Can you work these out from the model? Positions are in its coordinate system, mm. A direction names the side the tool comes from. Coordinates: 2 decimals unless noted, no trailing zeros. Order: outer loops, then holes, each group sorted by start corner. A loop starts at its lowest first (then second) coordinate and runs counter-clockwise, first axis right, second up. Notation, with made-up numbers: (-35, 33.5) -> (11, 33.5) arc R24 ccw to (11, 54.5) -> close; hole circle Ø1 at (86.25, 11.25). An arc over 180 degrees is marked (long way). Return JSON: item names as keys, results as strings. Group by question number.
1) For faces 1 (the flat face through (2, 50.8, 2)), 2 (the flat face through (2, 25.4, -46)), 3 (the flat face through (2, 50.8, -46)), 4 (the flat face through (2, 34.2, -22)), which set-ups out of +Z, -Z, +X, -X, +Y, -Y let a thin tool reach every point of the face, with its end or its side?
2) If we section it at A-A, the plane y = 66.7: Please give me the cut outline in (x, z) (3 decimals), then the cut area to 3 significant figures.
3) If we section it at D-D, the plane y = 10.5: Please give me the cut outline in (x, z) (3 decimals), then the cut area to 3 significant figures.
4) Thinking about a two-plate mould opening in Y: for faces 5 (the flat face through (2, 25.4, 2)), 6 (the flat face through (2, 49, -16.225)), 7 (the flat face through (2, 13, -44.45)), which applies, +Y half, -Y half, draft (parallel to the pull), parting line (faces both ways), or undercut?
5) If we section it at B-B, the plane x = 1.25: Please give me the cut outline in (y, z) (3 decimals), then the cut area to 3 significant figures.
6) If I drill on probe 1 along Y at (x, z) = (1.65, -27.5) (3 decimals); probe 2 along Z at (x, y) = (2.1, 52.5) (3 decimals); probe 3 along Z at (x, y) = (1.3, 48) (3 decimals), over which ranges is the centre line in solid material (lowest first)? Write a range as from..to.
7) If we section it at C-C, the plane y = 31.7: Please give me the cut outline in (x, z) (3 decimals).
8) For pin 1 (1.6 mm diameter, centred on x = 1.5, y = 74, fed in from +Z); pin 2 (12 mm diameter, centred on y = 46, z = -41, fed in from -X); pin 3 (1.6 mm diameter, centred on x = 1.5, z = 2, fed in from +Y); pin 4 (1.6 mm diameter, centred on x = 1, z = 2, fed in from -Y), each with a flat end and sliding along its axis, tell me the tip position at first contact or that it passes through.
Autodesk Inventor part; units mm, degrees
ref_plane "YZ Plane" through (0, 0, 0) normal (1, 0, 0) x (0, 1, 0)
ref_plane "XZ Plane" through (0, 0, 0) normal (0, 1, 0) x (-1, 0, 0)
ref_plane "XY Plane" through (0, 0, 0) normal (0, 0, 1) x (1, 0, 0)
sketch "Sketch1" plane through (0, 0, 0) normal (1, 0, 0) x (0, 1, 0)
  line L0 (0, 0) -> (76.2, 0)
  line L1 (76.2, 0) -> (76.2, -44.45)
  line L2 (76.2, -44.45) -> (0, -44.45)
  line L3 (0, -44.45) -> (0, 0)
  dimension "d0" = 76.2
  dimension "d1" = 44.45
extrude "Extrusion1" add sketch "Sketch1" along normal blind 3.175
sketch "Sketch2" plane through (3.175, 0, 0) normal (1, 0, 0) x (0, 0, -1)
  line L0 (44.45, 76.2) -> (0, 76.2)
  line L1 (13.7583, 76.2) -> (30.6917, 76.2)
  line L2 (30.6917, 76.2) -> (30.6917, 73.025)
  line L3 (30.6917, 73.025) -> (13.7583, 73.025)
  line L4 (13.7583, 73.025) -> (13.7583, 76.2)
  line L5 (0, 76.2) -> (0, 0)
  dimension "d4" = 16.9333
  dimension "d5" = 3.175
  dimension "d8" = 13.7583
extrude "Extrusion2" cut sketch "Sketch2" against normal blind 3.175
sketch "Sketch3" plane through (3.175, 0, 0) normal (1, 0, 0) x (0, 0, -1)
  line L0 (0, 76.2) -> (0, 0)
  line L1 (0, 0) -> (44.45, 0)
  line L2 (44.45, 0) -> (44.45, 76.2)
  line L3 (44.45, 50.8) -> (47.625, 50.8)
  line L4 (47.625, 50.8) -> (47.625, 25.4)
  line L5 (47.625, 25.4) -> (44.45, 25.4)
  line L6 (44.45, 25.4) -> (44.45, 50.8)
  line L7 (0, 50.8) -> (-3.175, 50.8)
  line L8 (-3.175, 50.8) -> (-3.175, 25.4)
  line L9 (-3.175, 25.4) -> (0, 25.4)
  line L10 (0, 25.4) -> (0, 50.8)
  dimension "d9" = 3.175
  dimension "d10" = 25.4
  dimension "d11" = 25.4
  dimension "d12" = 3.175
  dimension "d13" = 25.4
extrude "Extrusion3" add sketch "Sketch3" against normal blind 3.175
sketch "Sketch4" plane through (3.175, 0, 0) normal (1, 0, 0) x (0, 0, -1)
  line L0 (-3.175, 50.8) -> (-3.175, 25.4)
  line L1 (44.45, 76.2) -> (30.6917, 76.2)
  line L2 (16.225, 64.2) -> (28.225, 64.2)
  line L3 (28.225, 64.2) -> (28.225, 34.2)
  line L4 (28.225, 34.2) -> (16.225, 34.2)
  line L5 (16.225, 34.2) -> (16.225, 64.2)
  circle A0 centre (22.225, 66.7) radius 1.0541
  circle A1 centre (22.225, 31.7) radius 1.0541
  dimension "d16" = 12
  dimension "d17" = 30
  dimension "d19" = 19.4
  dimension "d20" = 12
  dimension "d21" = 2.1082
  dimension "d22" = 6
  dimension "d23" = 2.5
  dimension "d24" = 2.1082
  dimension "d25" = 6
  dimension "d26" = 2.5
extrude "Extrusion4" cut sketch "Sketch4" against normal blind 3.175
equation "\"d0\" = height"
equation "\"d1\" = depth - 2 * thick"
equation "\"d2\" = thick"
equation "\"d4\" = 0.333333 * depth"
equation "\"d5\" = thick"
equation "\"d8\" = 0.333333 * depth - thick"
equation "\"d6\" = thick"
equation "\"d9\" = thick"
equation "\"d10\" = 0.333333 * height"
equation "\"d11\" = 0.333333 * height"
equation "\"d12\" = thick"
equation "\"d13\" = 0.333333 * height"
equation "\"d14\" = thick"
equation "\"d16\" = servoWidth"
equation "\"d17\" = servoLength"
equation "\"d19\" = -0.5 * servoWidth + 0.5 * depth"
equation "\"d20\" = servoOffset"
equation "\"d21\" = servoHole"
equation "\"d22\" = 0.5 * servoWidth"
equation "\"d23\" = -0.5 * servoLength + 0.5 * servoDist"
equation "\"d24\" = servoHole"
equation "\"d25\" = 0.5 * servoWidth"
equation "\"d26\" = -0.5 * servoLength + 0.5 * servoDist"
equation "\"d27\" = thick"
equation "\"height\" = 76.2"
equation "\"thick\" = 3.175"
equation "\"depth\" = 50.8"
equation "\"servoLength\" = 30"
equation "\"servoWidth\" = 12"
equation "\"servoOffset\" = 12"
equation "\"servoDist\" = 35"
equation "\"servoHole\" = 2.1082"
properties part number "Side"
Result sheet:
{
 "1": {"face 1": "+Z, +X, -X, +Y", "face 2": "-Z, +X, -X, -Y", "face 3": "-Z, +X, -X, +Y", "face 4": "+X, -X"},
 "2": {"outline": "(0, -44.45) -> (3.175, -44.45) -> (3.175, -23.279) -> (0, -23.279) -> close; (0, -21.171) -> (3.175, -21.171) -> (3.175, 0) -> (0, 0) -> close", "area": "134 mm2"},
 "3": {"outline": "(0, -44.45) -> (3.175, -44.45) -> (3.175, 0) -> (0, 0) -> close", "area": "141 mm2"},
 "4": {"face 5": "-Y half", "face 6": "undercut", "face 7": "draft"},
 "5": {"outline": "(0, -44.45) -> (25.4, -44.45) -> (25.4, -47.625) -> (50.8, -47.625) -> (50.8, -44.45) -> (76.2, -44.45) -> (76.2, -30.692) -> (73.025, -30.692) -> (73.025, -13.758) -> (76.2, -13.758) -> (76.2, 0) -> (50.8, 0) -> (50.8, 3.175) -> (25.4, 3.175) -> (25.4, 0) -> (0, 0) -> close; hole circle Ø2.108 at (31.7, -22.225); hole (34.2, -28.225) -> (64.2, -28.225) -> (64.2, -16.225) -> (34.2, -16.225) -> close; hole circle Ø2.108 at (66.7, -22.225)", "area": "3,130 mm2"},
 "6": {"probe 1": "y = 0..34.2, 64.2..73.025", "probe 2": "z = -44.45..-28.225, -16.225..0", "probe 3": "z = -47.625..-28.225, -16.225..3.175"},
 "7": {"outline": "(0, -47.625) -> (3.175, -47.625) -> (3.175, -23.279) -> (0, -23.279) -> close; (0, -21.171) -> (3.175, -21.171) -> (3.175, 3.175) -> (0, 3.175) -> close"},
 "8": {"pin 1": "stops at z = 0", "pin 2": "stops at x = 0", "pin 3": "stops at y = 50.8", "pin 4": "stops at y = 25.4"}
}
